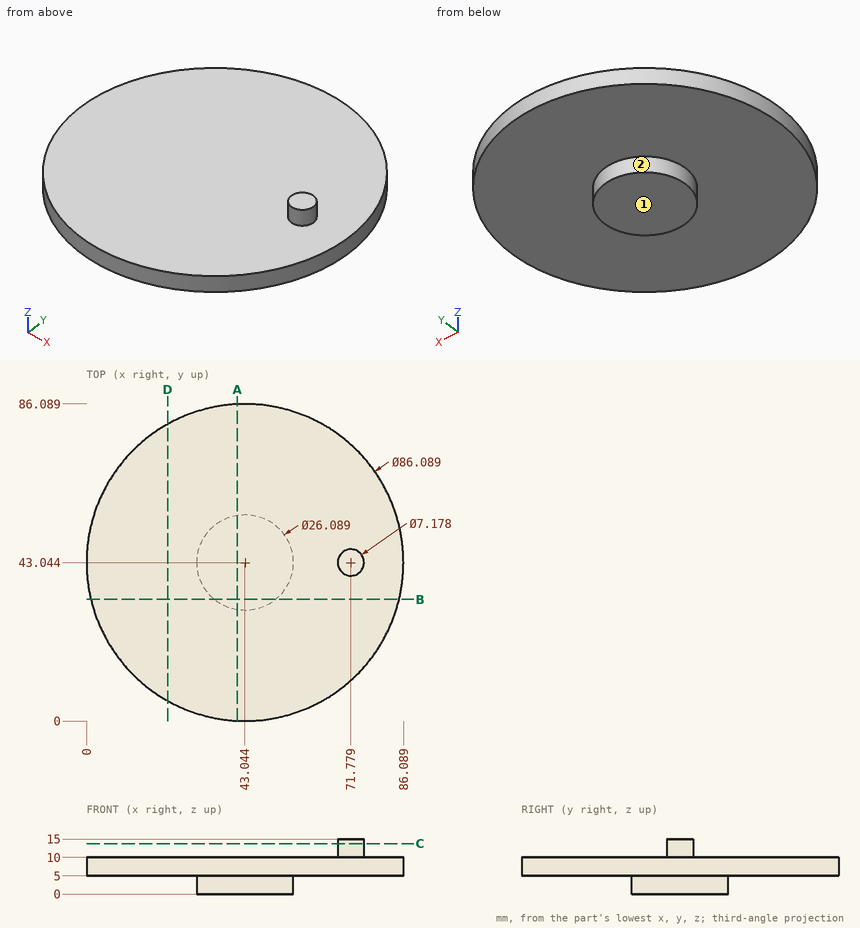
Design review of the part shown in the three views and the two pictorial views. Dimensions are in mm from the part's minimum x, y and z. A direction names the side the tool comes from. Give positions to 0.01 mm unless a question says otherwise; leave off trailing zeros. Write each loop counter-clockwise with the first axis right and the second up, starting at its lowest first coordinate (ties: lowest second). Pieces come first, ordered by that corner, then holes.
(1) Add section C-C (z = 13.75). Give the boundary of the cut face in (x, y) (1 decimal).
Checked values:
outline: circle Ø7.2 at (71.8, 43)
(2) Add section A-A (x = 41). Give the boundary of the cut face in (y, z).
Checked values:
outline: (0.05, 5) - (30.16, 5) - (30.16, 0) - (55.93, 0) - (55.93, 5) - (86.04, 5) - (86.04, 10) - (0.05, 10) - close
(3) Add section D-D (x = 22). Give the boundary of the cut face in (y, z) (1 decimal).
Checked values:
outline: (5.5, 5) - (80.6, 5) - (80.6, 10) - (5.5, 10) - close
(4) Clearance check with flat-ended pins moving along their axes: pin 1 Ø1.5 at (y, z) = (31, 12.5) entering from +X; pin 2 Ø1.5 at (x, z) = (65, 5) entering from -Y (1 decimal); pin 3 Ø3 at (x, z) = (30.5, 3) entering from -Y (1 decimal); pin 4 Ø1.5 at (y, z) = (10.5, 7.5) entering from -X. State where each tip first meets the part, or that it passes through.
Checked values:
pin 1: passes through
pin 2: stops at y = 5.6
pin 3: stops at y = 36.1
pin 4: stops at x = 14.03
(5) Tool access review of the marked faces 1 and 2: name each direction out of +Z, -Z, +X, -X, +Y, -Y from which nothing blocks a thin tool from reaching the whole face with its end or side.
Checked values:
face 1: -Z, +X, -X, +Y, -Y
face 2: -Z
(6) Add section B-B (y = 33). Give the boundary of the cut face in (x, z).
Checked values:
outline: (1.19, 5) - (34.72, 5) - (34.72, 0) - (51.37, 0) - (51.37, 5) - (84.9, 5) - (84.9, 10) - (1.19, 10) - close
(7) Wall thickness on line 1 along Z through (x, y) = (54, 39.5); line 2 along Z through (x, y) = (57, 28); line 3 along Y through (x, z) = (17.5, 6.25): over which ranges is each line inside the solid? List them lowest first.
Checked values:
line 1: z = 0 to 10
line 2: z = 5 to 10
line 3: y = 8.4 to 77.69
